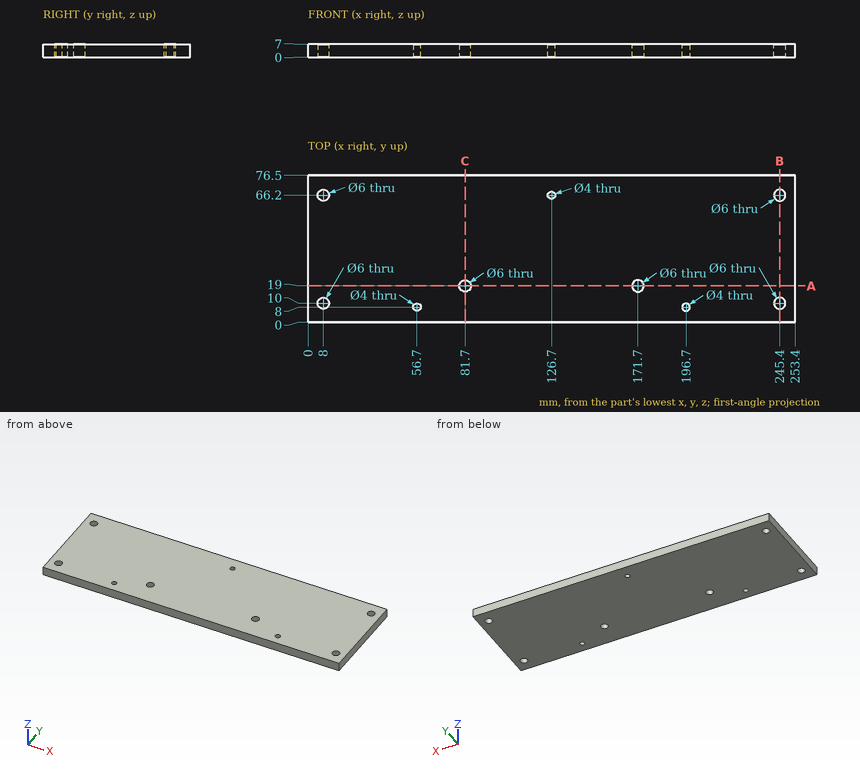
Source: three-view drawing plus pictorial views. Frame: mm from the lowest corner of the part. Give positions to 0.01 mm unless a question says otherwise; leave off trailing zeros. Loops run counter-clockwise (first coordinate to the right, second up) from the corner with the lowest first, then second, coordinate; pieces in that order, holes last.
1) Line query: L1, parallel to Y at x = 245.4, z = 5.5; L2, parallel to Y at x = 56.7, z = 5.75; L3, parallel to X at y = 12.5, z = 2.25. Output: solid intervals per line, ascending.
A:
L1: y = 0 to 7, 13 to 63.2, 69.2 to 76.5
L2: y = 0 to 6, 10 to 76.5
L3: x = 0 to 6.34, 9.66 to 243.74, 247.06 to 253.4
2) Section query C-C on x = 81.7. Return the cut outline in (y, z), and give its area (4 significant figures).
A:
outline: (0, 0) - (16, 0) - (16, 7) - (0, 7) - close; (22, 0) - (76.5, 0) - (76.5, 7) - (22, 7) - close
area: 493.5 mm2
3) Section query B-B on x = 245.4. Return the cut outline in (y, z).
A:
outline: (0, 0) - (7, 0) - (7, 7) - (0, 7) - close; (13, 0) - (63.2, 0) - (63.2, 7) - (13, 7) - close; (69.2, 0) - (76.5, 0) - (76.5, 7) - (69.2, 7) - close
4) Section query A-A on y = 19. Return the cut outline in (x, z).
A:
outline: (0, 0) - (78.7, 0) - (78.7, 7) - (0, 7) - close; (84.7, 0) - (168.7, 0) - (168.7, 7) - (84.7, 7) - close; (174.7, 0) - (253.4, 0) - (253.4, 7) - (174.7, 7) - close
